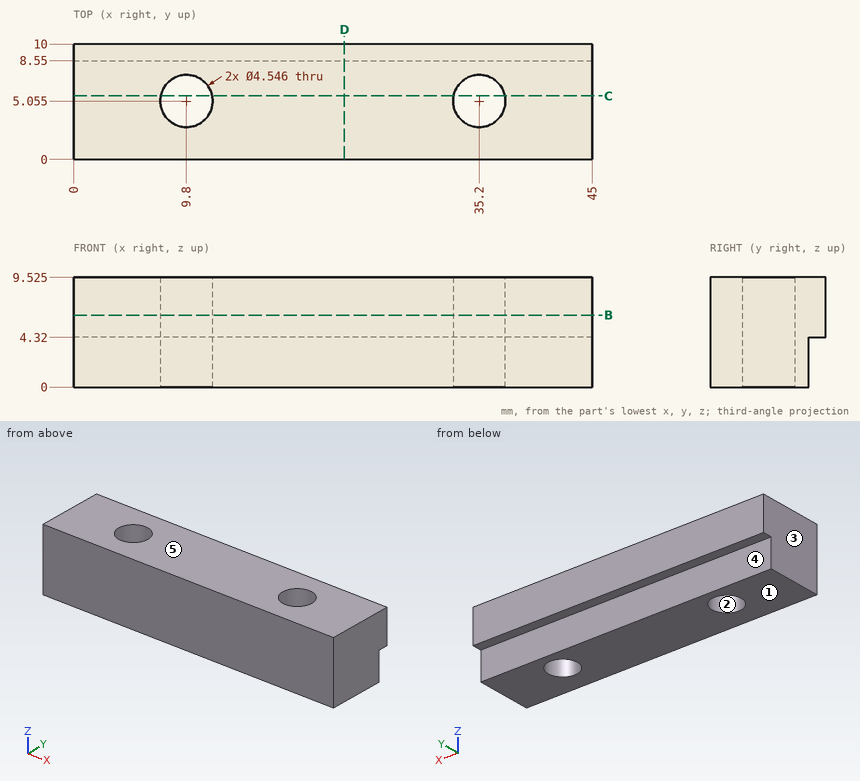
Part print with two shaded views. Sizes in mm from the minimum x, y, z corner. A direction names the side the tool comes from. Round coordinates to 2 decimals unless told otherwise and drop trailing zeros. Order: outer loops, then holes, each group sorted by start corner. A loop starts at its lowest first (then second) coordinate and runs counter-clockwise, first axis right, second up. Notation, with made-up numbers: M -14,70.5 L 4,70.5 A23 ccw 4,96.5 Z; hole C 50,16.5 d9. An arc over 180 degrees is marked long. Answer in a Markdown table with one row per item. Add a question column.
Q1. Cut at D-D on x = 23.5. Give the cut face in (y, z) (3 decimals).
Q2. 3-axis set-ups, long thin cutter, end or side, ignore diameter. For the marked faces 4 and 5: which of +Z, -Z, +X, -X, +Y, -Y reach the whole face in a straight line?
Q3. Cut at C-C on y = 5.5. Give the cut face in (x, z) (3 decimals).
Q4. Pin check, flat tips, straight feed: pin 1 (2 mm diameter, centred on x = 30.5, z = 1, fed in from +Y); pin 2 (2.5 mm diameter, centred on x = 35.2, y = 5.055, fed in from -Z). Stop position of each tip, or through.
Q5. Mould opens along X. For the marked faces 1, 2 and 3 say: +X half, -X half, draft (parallel to the pull), parting line (faces both ways), or undercut.
Q6. Wall check: L1, parallel to Y at x = 9.8, z = 3.75; L2, parallel to X at y = 3.25, z = 8.75; L3, parallel to X at y = 3, z = 4.75. Give the ranges that are in metal, low to high. Write a range as from..to.
Q7. Cut at B-B on z = 6.25. Give the cut face in (x, y) (1 decimal).
Established:
| question | item | result |
|---|---|---|
| 1 | outline | M 0,0 L 8.55,0 L 8.55,4.32 L 10,4.32 L 10,9.525 L 0,9.525 Z |
| 2 | face 4 | -Z, +X, -X, +Y |
| 2 | face 5 | +Z, +X, -X, +Y, -Y |
| 3 | outline | M 0,0 L 7.571,0 L 7.571,9.525 L 0,9.525 Z; M 12.029,0 L 32.971,0 L 32.971,9.525 L 12.029,9.525 Z; M 37.429,0 L 45,0 L 45,9.525 L 37.429,9.525 Z |
| 4 | pin 1 | stops at y = 8.55 |
| 4 | pin 2 | passes through |
| 5 | face 1 | draft |
| 5 | face 2 | undercut |
| 5 | face 3 | -X half |
| 6 | L1 | y = 0..2.78, 7.33..8.55 |
| 6 | L2 | x = 0..8.42, 11.18..33.82, 36.58..45 |
| 6 | L3 | x = 0..8.83, 10.77..34.23, 36.17..45 |
| 7 | outline | M 0,0 L 45,0 L 45,10 L 0,10 Z; hole C 9.8,5.1 d4.5; hole C 35.2,5.1 d4.5 |
